```python
from build123d import *

# Parameters (mm, degrees)
SKETCH_R   = 5
SKETCH_R_2 = 1.5
PAD_DEPTH  = 2


with BuildPart() as part:
    # Sketch → Pad (new body)
    with BuildSketch(Plane.XY):
        with BuildLine():
            ThreePointArc((-16.546601, 3.9), (-20.446601, 0), (-16.546601, -3.9))
            Line((-16.546601, -3.9), (-9.192388, -3.9))
            ThreePointArc((-3.9, -9.192388), (-5.450105, -5.450105), (-9.192388, -3.9))
            Line((-3.9, -16.546601), (-3.9, -9.192388))
            ThreePointArc((-3.9, -16.546601), (0, -20.446601), (3.9, -16.546601))
            Line((3.9, -16.546601), (3.9, -9.192388))
            ThreePointArc((9.192388, -3.9), (5.450105, -5.450105), (3.9, -9.192388))
            Line((16.546601, -3.9), (9.192388, -3.9))
            ThreePointArc((16.546601, -3.9), (20.446601, 0), (16.546601, 3.9))
            Line((16.546601, 3.9), (9.192388, 3.9))
            ThreePointArc((3.9, 9.192388), (5.450105, 5.450105), (9.192388, 3.9))
            Line((3.9, 16.546601), (3.9, 9.192388))
            ThreePointArc((3.9, 16.546601), (0, 20.446601), (-3.9, 16.546601))
            Line((-3.9, 16.546601), (-3.9, 9.192388))
            ThreePointArc((-9.192388, 3.9), (-5.450105, 5.450105), (-3.9, 9.192388))
            Line((-16.546601, 3.9), (-9.192388, 3.9))
        make_face()
        Circle(SKETCH_R, mode=Mode.SUBTRACT)
        with Locations((0, 16.5)):
            Circle(SKETCH_R_2, mode=Mode.SUBTRACT)
        with Locations((16.5, 0)):
            Circle(SKETCH_R_2, mode=Mode.SUBTRACT)
        with Locations((0, -16.5)):
            Circle(SKETCH_R_2, mode=Mode.SUBTRACT)
        with Locations((-16.5, 0)):
            Circle(SKETCH_R_2, mode=Mode.SUBTRACT)
    extrude(amount=-PAD_DEPTH)


solid = part.part
```
Geometry check sheet. Reference: the model listing, model coordinates, mm. A direction names the side the tool comes from. Give positions to 0.01 mm unless a question says otherwise; leave off trailing zeros. Loops run counter-clockwise (first coordinate to the right, second up) from the corner with the lowest first, then second, coordinate; pieces in that order, holes last. Notation, with made-up numbers: M 53.25,-12.5 L 104.25,-12.5 A14 ccw 104.25,-7.5 Z; hole C -7,25.25 d11. An arc over 180 degrees is marked long. Answer as CSV lines item,"result".
Item 1: Material ranges on line 1 (Y direction, x = 0, z = -0.85); line 2 (Y direction, x = 16.5, z = -0.65); line 3 (Y direction, x = 12.5, z = -0.6), recorded low to high.
Values:
line 1,"y = -20.45 to -18, -15 to -5, 5 to 15, 18 to 20.45"
line 2,"y = -3.9 to -1.5, 1.5 to 3.9"
line 3,"y = -3.9 to 3.9"
Item 2: Cross-section at B-B on z = -0.7. Record the cut outline in (x, y), and give its area (3 significant figures).
Values:
outline,"M -16.55,-3.9 L -9.19,-3.9 A5.29 cw -3.9,-9.19 L -3.9,-16.55 A3.9 ccw 3.9,-16.55 L 3.9,-9.19 A5.29 cw 9.19,-3.9 L 16.55,-3.9 A3.9 ccw 16.55,3.9 L 9.19,3.9 A5.29 cw 3.9,9.19 L 3.9,16.55 A3.9 ccw -3.9,16.55 L -3.9,9.19 A5.29 cw -9.19,3.9 L -16.55,3.9 A3.9 ccw Z; hole C -16.5,0 d3; hole C 0,0 d10; hole C 0,-16.5 d3; hole C 0,16.5 d3; hole C 16.5,0 d3"
area,"468 mm²"
Item 3: Cross-section at C-C on y = 15.5. Record the cut outline in (x, z).
Values:
outline,"M -3.9,-2 L -1.12,-2 L -1.12,0 L -3.9,0 Z; M 1.12,-2 L 3.9,-2 L 3.9,0 L 1.12,0 Z"
Item 4: Release check for a two-part mould opening along X. For faces 5 (the cylindrical face through (0.086, 20.446, -0.986)), 6 (the flat face through (-13, 3.9, -1)), 7 (the cylindrical face through (-1.11, 17.51, -0.99)), 8 (the cylindrical face through (20.446, -0.086, -0.986)) record: pulls with the +X half, pulls with the -X half, needs draft (parallel to the pull), parting line crosses it, or undercut.
Values:
face 5,"parting line crosses it"
face 6,"needs draft"
face 7,"undercut"
face 8,"pulls with the +X half"
Item 5: Cross-section at D-D on x = 6. Record the cut outline in (y, z), and give its area (3 significant figures).
Values:
outline,"M -4.97,-2 L 4.97,-2 L 4.97,0 L -4.97,0 Z"
area,"19.9 mm²"
Item 6: Depth check by flat-ended pin: P1, Ø1, axis at x = 14.5, z = -1.5, coming from the +Y side; P2, Ø0.6, axis at x = -11.5, z = -1, coming from the -Y side. Enter the tip coordinate at first touch or a pass-through.
Values:
P1,"stops at y = 3.9"
P2,"stops at y = -3.9"
Item 7: Cross-section at A-A on x = 0. Record the cut outline in (y, z), and give its area (3 significant figures).
Values:
outline,"M -20.45,-2 L -18,-2 L -18,0 L -20.45,0 Z; M -15,-2 L -5,-2 L -5,0 L -15,0 Z; M 5,-2 L 15,-2 L 15,0 L 5,0 Z; M 18,-2 L 20.45,-2 L 20.45,0 L 18,0 Z"
area,"49.8 mm²"
Item 8: Access from +Z, -Z, +X, -X, +Y, -Y to the whole of each face (thin tool, end or side, straight path). Record for faces 1 (the flat face through (3.9, -13, -1)), 2 (the flat face through (-13, -3.9, -1)), 3 (the flat face through (-3.9, 13, -1)), 4 (the flat face through (3.9, 13, -1)).
Values:
face 1,"+Z, -Z, +X, -Y"
face 2,"+Z, -Z, -X, -Y"
face 3,"+Z, -Z, -X, +Y"
face 4,"+Z, -Z, +X, +Y"
